Autodesk Inventor part; units mm, degrees
ref_plane "YZ Plane" through (0, 0, 0) normal (1, 0, 0) x (0, 1, 0)
ref_plane "XZ Plane" through (0, 0, 0) normal (0, 1, 0) x (-1, 0, 0)
ref_plane "XY Plane" through (0, 0, 0) normal (0, 0, 1) x (1, 0, 0)
sketch "Sketch1" plane through (0, 0, 0) normal (0, 0, 1) x (1, 0, 0)
  line L0 (3.25, -3.75) -> (-3.25, -3.75)
  line L1 (-3.75, -3.25) -> (-3.75, 3.25)
  line L2 (-3.25, 3.75) -> (3.25, 3.75)
  line L3 (3.75, 3.25) -> (3.75, -3.25)
  line L4 (3.75, -3.75) -> (-3.75, 3.75) construction
  line L5 (-3.75, -3.75) -> (3.75, 3.75) construction
  arc A0 (-3.25, 3.75) -> (-3.75, 3.25) centre (-3.25, 3.25) ccw
  arc A1 (-3.75, -3.25) -> (-3.25, -3.75) centre (-3.25, -3.25) ccw
  arc A2 (3.25, -3.75) -> (3.75, -3.25) centre (3.25, -3.25) ccw
  arc A3 (3.75, 3.25) -> (3.25, 3.75) centre (3.25, 3.25) ccw
  point P0 (0, 0)
  dimension "d0" = 7.5
  dimension "d1" = 0.5
extrude "Extrusion1" add sketch "Sketch1" along normal mid plane 3.02
sketch "Sketch2" plane through (0, 0, -1.51) normal (0, 0, -1) x (-1, 0, 0)
  line L0 (2.96, -3) -> (1.56, -3)
  line L1 (1.56, -3) -> (1.56, 3)
  line L2 (1.56, 3) -> (2.96, 3)
  line L3 (2.96, 3) -> (2.96, -3)
  line L4 (-1.56, -3) -> (-2.96, -3)
  line L5 (-2.96, -3) -> (-2.96, 3)
  line L6 (-2.96, 3) -> (-1.56, 3)
  line L7 (-1.56, 3) -> (-1.56, -3)
  line L8 (0, -3) -> (0, 3) construction
  point P0 (0, 0)
  point P1 (0, 0)
  dimension "d4" = 1.4
  dimension "d5" = 6
  dimension "d6" = 3.12
extrude "Extrusion2" add sketch "Sketch2" along normal blind 0.08
sketch "Sketch3" plane through (0, 0, 1.51) normal (0, 0, 1) x (1, 0, 0)
  line L0 (2.75, 2.5) -> (2.5, 2.5)
  line L1 (2.5, 2.5) -> (2.5, -2.5)
  line L2 (2.5, -2.5) -> (2.75, -2.5)
  line L3 (2.75, -2.5) -> (2.75, 2.5)
  line L4 (-2.5, 2.5) -> (-2.5, -2.5) construction
  spline S0 degree 4 poles (1.3361, 0.4296) (1.5722, 0.2536) (1.6111, 0.0081) (1.8752, -0.3041) (1.3349, -0.7643) (0.9016, -0.6061) (0.6086, -0.3512) (0.6279, 0.0301) (0.8528, 0.1857) (1.2221, 0.0137) (1.0663, -0.2096) (0.9971, -0.1716) (0.8339, -0.0827) (0.9372, -0.3475) (1.124, -0.4244) (1.5104, -0.4795) (1.4218, 0.1865) (0.9203, 0.4463) (0.2397, 0.5724) (-0.0703, -0.2361) (0.2655, -0.4716) (0.366, -0.6909) (0.4591, -0.7727) knots 0 0 0 0 0 0.123761 0.174234 0.226685 0.279962 0.33014 0.377129 0.419078 0.455262 0.487036 0.514913 0.545248 0.580512 0.622872 0.674906 0.733244 0.796807 0.860625 0.919671 1 1 1 1 1
  line L5 (0.3021, -0.6347) -> (0.6161, -0.9108) construction
  arc A0 (0.3672, -0.6474) -> (0.5952, -0.8479) centre (0.698, -0.5011) ccw construction
  spline S1 degree 4 poles (1.3361, 0.4296) (1.1748, 0.5523) (0.7861, 0.8379) (-0.1178, 0.7487) (-0.2762, -0.1647) (0.0057, -0.6403) (0.1538, -0.7727) knots 0 0 0 0 0 0.46045 0.670358 1 1 1 1 1
  line L6 (-0.0024, -0.6331) -> (0.3101, -0.9124) construction
  arc A1 (0.0518, -0.6477) -> (0.2895, -0.8602) centre (0.4983, -0.3874) ccw construction
  line L7 (0.4591, -0.7727) -> (0.1538, -0.7727)
  line L8 (1.4819, -0.2272) -> (1.2942, 0.2269) construction
  arc A2 (1.4343, -0.1846) -> (1.2905, 0.1631) centre (0.7871, -0.2485) ccw construction
  line L9 (-2.5, 0.7834) -> (-2.5, 1.7741)
  line L10 (-2.5, 1.7741) -> (-2.2387, 1.7741)
  line L11 (-2.2387, 1.7741) -> (-2.2387, 1.4581)
  line L12 (-2.2387, 1.4581) -> (-1.4449, 1.4581)
  line L13 (-1.4449, 1.4581) -> (-1.4449, 1.7741)
  line L14 (-1.4449, 1.7741) -> (-1.2006, 1.7741)
  spline S2 degree 2 poles (-1.2006, 1.7741) (-1.2006, 1.7048) (-1.1823, 1.5675) (-1.1629, 1.5261) knots 0 0 0 1 2 2 2
  spline S3 degree 2 poles (-1.1629, 1.5261) (-1.1386, 1.4787) (-1.0571, 1.4252) (-0.9964, 1.4204) knots 0 0 0 1 2 2 2
  line L15 (-0.9964, 1.4204) -> (-0.9964, 1.0922)
  line L16 (-0.9964, 1.0922) -> (-2.2387, 1.0922)
  line L17 (-2.2387, 1.0922) -> (-2.2387, 0.7834)
  line L18 (-2.2387, 0.7834) -> (-2.5, 0.7834)
  spline S4 degree 2 poles (-1.75, -0.578) (-1.9445, -0.578) (-2.2362, -0.516) (-2.3347, -0.4467) knots 0 0 0 1 2 2 2
  spline S5 degree 2 poles (-2.3347, -0.4467) (-2.4319, -0.3786) (-2.5316, -0.1586) (-2.5316, -0.0006) knots 0 0 0 1 2 2 2
  spline S6 degree 2 poles (-2.5316, -0.0006) (-2.5316, 0.1586) (-2.4319, 0.3774) (-2.3323, 0.4467) knots 0 0 0 1 2 2 2
  spline S7 degree 2 poles (-2.3323, 0.4467) (-2.2338, 0.516) (-1.9445, 0.578) (-1.75, 0.578) knots 0 0 0 1 2 2 2
  spline S8 degree 2 poles (-1.75, 0.578) (-1.5506, 0.578) (-1.2686, 0.516) (-1.1665, 0.4455) knots 0 0 0 1 2 2 2
  spline S9 degree 2 poles (-1.1665, 0.4455) (-1.0669, 0.375) (-0.9696, 0.1526) (-0.9696, -0.0006) knots 0 0 0 1 2 2 2
  spline S10 degree 2 poles (-0.9696, -0.0006) (-0.9696, -0.1623) (-1.0717, -0.3786) (-1.1726, -0.4479) knots 0 0 0 1 2 2 2
  spline S11 degree 2 poles (-1.1726, -0.4479) (-1.2711, -0.516) (-1.5616, -0.578) (-1.75, -0.578) knots 0 0 0 1 2 2 2
  spline S12 degree 2 poles (-1.75, -0.2) (-1.4716, -0.2) (-1.2468, -0.1088) (-1.2468, -0.0006) knots 0 0 0 1 2 2 2
  spline S13 degree 2 poles (-1.2468, -0.0006) (-1.2468, 0.1076) (-1.4716, 0.2) (-1.7512, 0.2) knots 0 0 0 1 2 2 2
  spline S14 degree 2 poles (-1.7512, 0.2) (-2.0259, 0.2) (-2.2545, 0.1076) (-2.2545, -0.0006) knots 0 0 0 1 2 2 2
  spline S15 degree 2 poles (-2.2545, -0.0006) (-2.2545, -0.1076) (-2.0259, -0.2) (-1.75, -0.2) knots 0 0 0 1 2 2 2
  line L19 (-2.5, -1.9115) -> (-2.5, -0.809)
  line L20 (-2.5, -0.809) -> (-2.2557, -0.809)
  spline S16 degree 2 poles (-2.2557, -0.809) (-2.1438, -0.9487) (-1.9469, -1.1724) (-1.8582, -1.2563) knots 0 0 0 1 2 2 2
  spline S17 degree 2 poles (-1.8582, -1.2563) (-1.7427, -1.3669) (-1.5665, -1.4654) (-1.4741, -1.4654) knots 0 0 0 1 2 2 2
  spline S18 degree 2 poles (-1.4741, -1.4654) (-1.3695, -1.4654) (-1.2577, -1.3402) (-1.2577, -1.2283) knots 0 0 0 1 2 2 2
  spline S19 degree 2 poles (-1.2577, -1.2283) (-1.2577, -1.1712) (-1.2857, -1.0691) (-1.3075, -1.0168) knots 0 0 0 1 2 2 2
  spline S20 degree 2 poles (-1.3075, -1.0168) (-1.3306, -0.9658) (-1.3793, -0.8928) (-1.3914, -0.8746) knots 0 0 0 1 2 2 2
  line L21 (-1.3914, -0.8746) -> (-1.3914, -0.8454)
  line L22 (-1.3914, -0.8454) -> (-1.0644, -0.8454)
  spline S21 degree 2 poles (-1.0644, -0.8454) (-1.034, -0.9086) (-0.9708, -1.1785) (-0.9708, -1.3037) knots 0 0 0 1 2 2 2
  spline S22 degree 2 poles (-0.9708, -1.3037) (-0.9708, -1.5711) (-1.2091, -1.8458) (-1.4242, -1.8458) knots 0 0 0 1 2 2 2
  spline S23 degree 2 poles (-1.4242, -1.8458) (-1.5567, -1.8458) (-1.812, -1.7206) (-1.9579, -1.576) knots 0 0 0 1 2 2 2
  spline S24 degree 2 poles (-1.9579, -1.576) (-2.0478, -1.4848) (-2.1876, -1.3134) (-2.2168, -1.2757) knots 0 0 0 1 2 2 2
  line L23 (-2.2168, -1.2757) -> (-2.2168, -1.9115)
  line L24 (-2.2168, -1.9115) -> (-2.5, -1.9115)
  point P0 (0, 0)
  point P1 (-2.5, 0)
  point P2 (2.5, 0)
  point P3 (1.5897, 0.1222)
  point P4 (1.6836, -0.1324)
  point P5 (1.6666, -0.392)
  point P6 (1.348, -0.657)
  point P7 (0.9064, -0.5696)
  point P8 (0.6595, -0.2864)
  point P9 (0.6874, 0.0129)
  point P10 (0.9152, 0.1153)
  point P11 (1.131, -0.0524)
  point P12 (1.0559, -0.1747)
  point P13 (0.9784, -0.1613)
  point P14 (0.8944, -0.1391)
  point P15 (0.915, -0.2539)
  point P16 (1.1067, -0.4034)
  point P17 (1.3658, -0.3897)
  point P18 (1.3881, -0.0001)
  point P19 (0.911, 0.405)
  point P20 (0.2939, 0.3734)
  point P21 (0.0837, -0.1519)
  point P22 (0.2608, -0.5163)
  point P23 (1.0376, 0.6174)
  point P24 (0.5316, 0.7174)
  point P25 (0.0302, 0.4881)
  point P26 (-0.1564, -0.1329)
  dimension "d9" = 5
  dimension "d10" = 0.25
  dimension "d11" = 2.5
  dimension "d12" = 2.5
extrude "Extrusion3" add sketch "Sketch3" along normal blind 0.01
properties part number "Inductor_7575" material "Steel, Carbon"
Can you work these out from the model? Positions are in its coordinate system, mm. Round coordinates to 2 decimals unless told otherwise and drop trailing zeros. Loops run counter-clockwise (first coordinate to the right, second up) from the corner with the lowest first, then second, coordinate; pieces in that order, holes last. Notation, with made-up numbers: (56, 15.25) -> (61, 15.25) arc R19 ccw to (61, 49.25) -> close; hole circle Ø10 at (51, 34.5). An arc over 180 degrees is marked (long way). Answer in a Markdown table with one row per item.
Item 1: We'd pull the mould along X, two halves only. Please class faces 1 (the flat face through (0, 1, 1.51)), 2 (the flat face through (3.75, 0, 0)), 3 (the flat face through (-2, 0, -1.59)), 4 (the flat face through (0, 0, -1.51)): released by +X, released by -X, zero draft, split by the parting line, or undercut.
Answer block:
| item | result |
|---|---|
| face 1 | undercut |
| face 2 | released by +X |
| face 3 | zero draft |
| face 4 | undercut |
Item 2: If I drill on probe 1 along Z at (x, y) = (-1.25, -1.5); probe 2 along Z at (x, y) = (-2.25, -2); probe 3 along X at (y, z) = (-3.5, 0), over which ranges is the centre line in solid material (lowest first)?
Answer block:
| item | result |
|---|---|
| probe 1 | -1.51 to 1.52 |
| probe 2 | -1.59 to 1.51 |
| probe 3 | -3.68 to 3.68 |
Item 3: Suppose I cut it at B-B, the plane x = -0.5. List the corners of the cut face in (y, z) for me, plus the area to 4 significant figures.
Answer block:
| item | result |
|---|---|
| outline | (-3.75, -1.51) -> (3.75, -1.51) -> (3.75, 1.51) -> (-3.75, 1.51) -> close |
| area | 22.65 mm² |
Item 4: Suppose I cut it at C-C, the plane x = -3.5. List the corners of the cut face in (y, z) for me.
Answer block:
| item | result |
|---|---|
| outline | (-3.68, -1.51) -> (3.68, -1.51) -> (3.68, 1.51) -> (-3.68, 1.51) -> close |
